For this review, take the finished solid that the model builds, in its own axes (mm). A direction names the side the tool comes from. Coordinates: 2 decimals unless noted, no trailing zeros. Order: outer loops, then holes, each group sorted by start corner. A loop starts at its lowest first (then second) coordinate and runs counter-clockwise, first axis right, second up. Notation, with made-up numbers: (74.5, -30) -> (81.5, -30) arc R10 ccw to (81.5, -25) -> close; hole circle Ø9 at (-26.5, 39.25). An arc over 180 degrees is marked (long way). Write item = value, one per line. Start each with the question number.
1) Consider section C-C on z = -5. Give the boundary of the cut face in (x, y), and give its area (3 significant figures).
2) Insertion check: pin 1 Ø3 at (y, z) = (-4.5, -6.5) entering from +X; pin 2 Ø6.5 at (x, y) = (3.5, 3) entering from +Z; pin 3 Ø3 at (x, y) = (4.5, 2.5) entering from -Z. Each pin has a flat end and moves straight along its axis. Give the tip position at first contact, or say it passes through.
3) Consider section D-D on x = -5.75. Give the boundary of the cut face in (y, z), and give its area (3 significant figures).
4) Consider section B-B on y = 0. Give the boundary of the cut face in (x, z), and give its area (3 significant figures).
5) Consider section A-A on x = 0. Give the boundary of the cut face in (y, z), and give its area (3 significant figures).
6) Draft analysis for pull direction X (two halves, no side actions). For faces 5 (the face through (-6, -10, 7)), 6 (the face through (0, 2, 4)), state which applies: +X half, -X half, draft (parallel to the pull), parting line (faces both ways), or undercut.
7) Wall thickness on probe 1 along Y at (x, z) = (0, 2.5); probe 2 along Y at (x, z) = (0, 5.5); probe 3 along Y at (x, z) = (0, 1.8): over which ranges is each line inside the solid? List them lowest first. Write a range as [from, to].
8) Machinability: for faces 1 (the face through (2.395, -10.787, -12.675)), 2 (the face through (2.5, -0.1, 3)), 3 (the face through (6, -10, -25)), 4 (the face through (1, 0, 2)), which of the approach directions +Z, -Z, +X, -X, +Y, -Y give a long, thin tool a straight path to every point of the face, cutting with its end or side? Answer none if there is none.
from build123d import *

# Parameters (mm, degrees)
SKETCH_1_R          = 13
SKETCH_1_R_2        = 11
EXTRUDE_1_DEPTH     = 7
SKETCH_3_R          = 13
EXTRUDE_2_DEPTH     = 2
CUT_EXTRUDE_1_REACH = 21.672
SKETCH_7_R          = 2.5
EXTRUDE_3_DEPTH     = 2
EXTRUDE_START       = 27
SKETCH_8_R          = 13
SKETCH_8_R_2        = 11
EXTRUDE_4_DEPTH     = 27
SKETCH_10_R         = 11.05
CUT_EXTRUDE_2_DEPTH = 27
CUT_EXTRUDE_START   = -5
SKETCH_11_R         = 11.05
SKETCH_11_R_2       = 2.5
CUT_EXTRUDE_3_DEPTH = 5
SKETCH_12_R         = 14.847927408
CUT_EXTRUDE_4_DEPTH = 2


with BuildPart() as part:
    # 草图1 → 凸台-拉伸1 (new body)
    with BuildSketch(Plane.XY):
        Circle(SKETCH_1_R)
        Circle(SKETCH_1_R_2, mode=Mode.SUBTRACT)
    extrude(amount=EXTRUDE_1_DEPTH)

    # 草图3 → 凸台-拉伸2 (add)
    with BuildSketch(Plane(origin=(0, 0, 0), x_dir=(-1, 0, 0), z_dir=(0, 0, -1))):
        with Locations(Location((0, 0, 0), (0, 0, 180))):
            Circle(SKETCH_3_R)
    extrude(amount=-EXTRUDE_2_DEPTH)

    # 草图6 → 切除-拉伸1 (cut, up to next)
    with BuildSketch(Plane(origin=(0, 0, 0), x_dir=(-1, 0, 0), z_dir=(0, 0, -1)), mode=Mode.PRIVATE) as cut_extrude_1_sk1:
        with BuildLine():
            Line((-1, -1.118033989), (-1, 1.118033989))
            ThreePointArc((-1, 1.118033989), (1.5, 0), (-1, -1.118033989))
        make_face()
    cut_extrude_1_tool1 = extrude(cut_extrude_1_sk1.sketch, amount=-CUT_EXTRUDE_1_REACH, mode=Mode.PRIVATE) & part.part
    add(cut_extrude_1_tool1.solids().sort_by_distance((-0.148024, 0, 0))[0], mode=Mode.SUBTRACT)

    # 草图7 → 凸台-拉伸3 (add)
    with BuildSketch(Plane.XY.offset(2)):
        with Locations(Location((0, 0, 0), (0, 0, 180))):
            Circle(SKETCH_7_R)
        with BuildLine():
            Line((1, -1.118033989), (1, 1.118033989))
            ThreePointArc((1, 1.118033989), (-1.5, 0), (1, -1.118033989))
        make_face(mode=Mode.SUBTRACT)
    extrude(amount=EXTRUDE_3_DEPTH)

    # 草图8 → 凸台-拉伸4 (add)
    with BuildSketch(Plane(origin=(0, 0, 0), x_dir=(-1, 0, 0), z_dir=(0, 0, -1)).offset(EXTRUDE_START)):
        Circle(SKETCH_8_R)
        Circle(SKETCH_8_R_2, mode=Mode.SUBTRACT)
    extrude(amount=-EXTRUDE_4_DEPTH)

    # 草图10 → 切除-拉伸2 (cut)
    with BuildSketch(Plane(origin=(0, 0, -27), x_dir=(-1, 0, 0), z_dir=(0, 0, -1))):
        Circle(SKETCH_10_R)
    extrude(amount=-CUT_EXTRUDE_2_DEPTH, mode=Mode.SUBTRACT)

    # 草图11 → 切除-拉伸3 (cut)
    with BuildSketch(Plane.XY.offset(7).offset(CUT_EXTRUDE_START)):
        with Locations(Location((0, 0, 0), (0, 0, 180))):
            Circle(SKETCH_11_R)
        with Locations(Location((0, 0, 0), (0, 0, 180))):
            Circle(SKETCH_11_R_2, mode=Mode.SUBTRACT)
    extrude(amount=CUT_EXTRUDE_3_DEPTH, mode=Mode.SUBTRACT)

    # 草图12 → 切除-拉伸4 (cut)
    with BuildSketch(Plane(origin=(0, 0, -27), x_dir=(-1, 0, 0), z_dir=(0, 0, -1))):
        Circle(SKETCH_12_R)
    extrude(amount=-CUT_EXTRUDE_4_DEPTH, mode=Mode.SUBTRACT)


solid = part.part
Answer sheet:
q1.outline = circle Ø26 at (0, 0); hole circle Ø22.1 at (0, 0)
q1.area = 147 mm2
q2.pin_1 = 12.65
q2.pin_2 = 4
q2.pin_3 = 0
q3.outline = (-11.66, -25) -> (-9.44, -25) -> (-9.44, 0) -> (9.44, 0) -> (9.44, -25) -> (11.66, -25) -> (11.66, 7) -> (9.44, 7) -> (9.44, 2) -> (-9.44, 2) -> (-9.44, 7) -> (-11.66, 7) -> close
q3.area = 180 mm2
q4.outline = (-13, -25) -> (-11.05, -25) -> (-11.05, 0) -> (-1.5, 0) -> (-1.5, 4) -> (-2.5, 4) -> (-2.5, 2) -> (-11.05, 2) -> (-11.05, 7) -> (-13, 7) -> close; (1, 0) -> (11.05, 0) -> (11.05, -25) -> (13, -25) -> (13, 7) -> (11.05, 7) -> (11.05, 2) -> (2.5, 2) -> (2.5, 4) -> (1, 4) -> close
q4.area = 169 mm2
q5.outline = (-13, -25) -> (-11.05, -25) -> (-11.05, 0) -> (-1.5, 0) -> (-1.5, 4) -> (-2.5, 4) -> (-2.5, 2) -> (-11.05, 2) -> (-11.05, 7) -> (-13, 7) -> close; (1.5, 0) -> (11.05, 0) -> (11.05, -25) -> (13, -25) -> (13, 7) -> (11.05, 7) -> (11.05, 2) -> (2.5, 2) -> (2.5, 4) -> (1.5, 4) -> close
q5.area = 167 mm2
q6.face_5 = draft
q6.face_6 = undercut
q7.probe_1 = [-13, -11.05], [-2.5, -1.5], [1.5, 2.5], [11.05, 13]
q7.probe_2 = [-13, -11.05], [11.05, 13]
q7.probe_3 = [-13, -1.5], [1.5, 13]
q8.face_1 = -Z
q8.face_2 = +Z
q8.face_3 = -Z, +X, -X, +Y, -Y
q8.face_4 = +Z, -Z
